Can you work these out from the drawing? Everything is in mm from the part's minimum corner. A direction names the side the tool comes from. Round coordinates to 2 decimals unless told otherwise and drop trailing zeros. Write each loop counter-clockwise with the first axis right and the second up, starting at its lowest first coordinate (ties: lowest second). Pieces come first, ordered by that corner, then holes. Notation, with made-up numbers: M 80.5,71 L 130.5,71 A21 cw 130.5,103 Z; hole C 28,37.25 d2. An arc over 180 degrees is marked long. Use one line per item in the form item = value. Start each with the question number.
Q1. I want a section at B-B on x = 6.75. List the corners of the cut face in (y, z) for me.
Q2. I'm going to push flat-ended pins straight in: pin 1 Ø1.2 at (x, z) = (14.5, 7) entering from +Y (3 decimals); pin 2 Ø0.7 at (x, z) = (15, 11.5) entering from -Y (3 decimals); pin 3 Ø3 at (x, y) = (13.5, 18.5) entering from +Z. Where does each tip first touch, or does it pass through?
Q3. We'd pull the mould along X, two halves only. Please class the marked faces 1, 2, 3 and 4: +X half, -X half, draft (parallel to the pull), parting line (faces both ways), or undercut.
Q4. I want a section at D-D on z = 2.25. List the corners of the cut face in (x, y) for me (3 decimals).
Q5. I want a section at A-A on y = 11.5. List the corners of the cut face in (x, z) for me, and give its area (3 significant figures).
Q6. I want a section at C-C on y = 31. List the corners of the cut face in (x, z) for me.
Q7. For the marked faces 5, 6, 7 and 8, which set-ups out of +Z, -Z, +X, -X, +Y, -Y let a thin tool reach every point of the face, with its end or its side?
Q8. I need wall thicknesses on line 1 along X through (y, z) = (12, 2); line 2 along Y through (x, z) = (5.5, 2.25); line 3 along Y through (x, z) = (14.25, 7.5) (3 decimals). Which ranges of each line are inside material? Lowest first, please. Write a range as from..to.
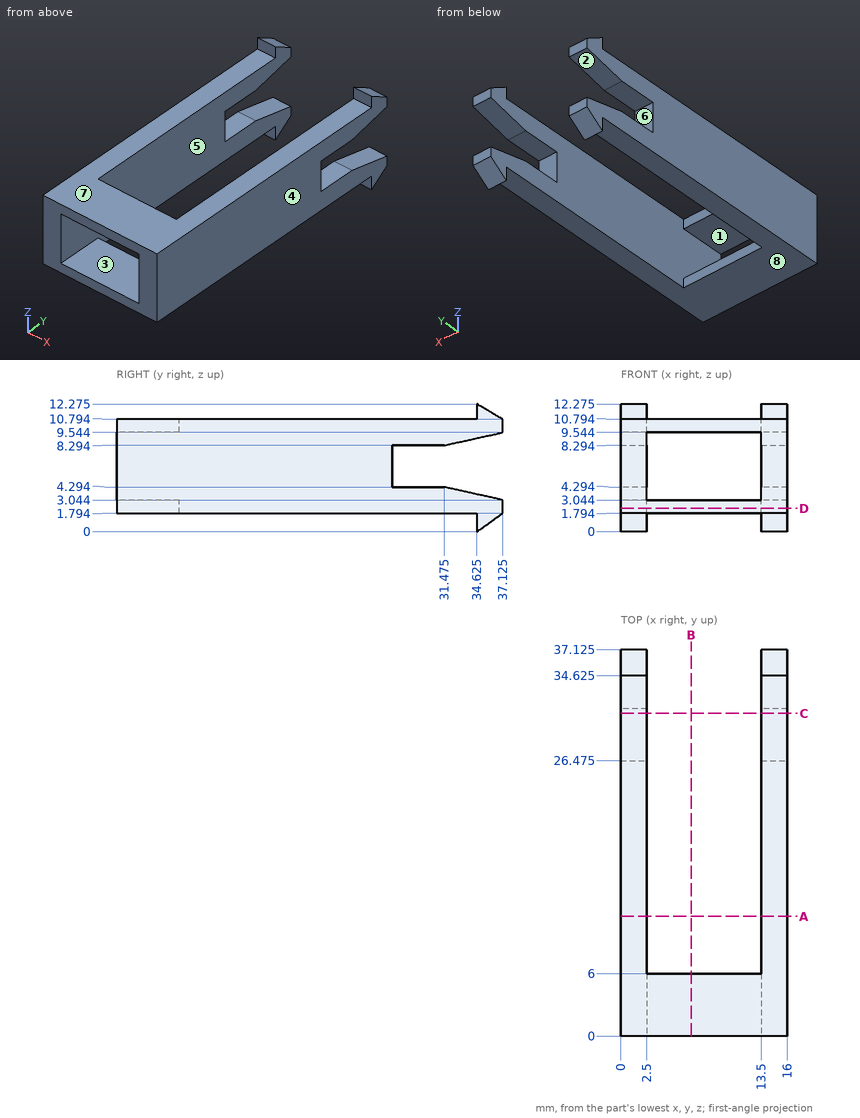
Reported:
q1.outline = M 0,1.79 L 6,1.79 L 6,3.04 L 0,3.04 Z; M 0,9.54 L 6,9.54 L 6,10.79 L 0,10.79 Z
q2.pin_1 = 26.475
q2.pin_2 = 34.625
q2.pin_3 = 10.79
q3.face_1 = undercut
q3.face_2 = draft
q3.face_3 = undercut
q3.face_4 = +X half
q4.outline = M 0,0 L 16,0 L 16,37.125 L 13.5,37.125 L 13.5,6 L 2.5,6 L 2.5,37.125 L 0,37.125 Z
q5.outline = M 0,1.79 L 2.5,1.79 L 2.5,10.79 L 0,10.79 Z; M 13.5,1.79 L 16,1.79 L 16,10.79 L 13.5,10.79 Z
q5.area = 45.0 mm^2
q6.outline = M 0,1.79 L 2.5,1.79 L 2.5,4.29 L 0,4.29 Z; M 0,8.29 L 2.5,8.29 L 2.5,10.79 L 0,10.79 Z; M 13.5,1.79 L 16,1.79 L 16,4.29 L 13.5,4.29 Z; M 13.5,8.29 L 16,8.29 L 16,10.79 L 13.5,10.79 Z
q7.face_5 = +Y
q7.face_6 = +X, -X, +Y
q7.face_7 = +Z, +X, -X, -Y
q7.face_8 = -Z, +X, -X, -Y
q8.line_1 = 0..2.5, 13.5..16
q8.line_2 = 0..6
q8.line_3 = 0..26.475
